from build123d import *

# Parameters (mm, degrees)
SKETCH_1_W             = 30
SKETCH_1_H             = 20
SKETCH_1_R             = 1.5
EXTRUDE_1_DEPTH        = 5
CUT_EXTRUDE_1_DEPTH    = 19.708286934
PATTERN_LINEAR_1_COUNT = 10
PATTERN_LINEAR_1_PITCH = 3


with BuildPart() as part:
    # 草图1 → 凸台-拉伸1 (new body)
    with BuildSketch(Plane(origin=(0, 0, 0), x_dir=(1, 0, 0), z_dir=(0, 1, 0))):
        Rectangle(SKETCH_1_W, SKETCH_1_H)
        with Locations(Location((-10, 7, 0), (0, 0, 270))):
            Circle(SKETCH_1_R, mode=Mode.SUBTRACT)
        with Locations(Location((10, 7, 0), (0, 0, 90))):
            Circle(SKETCH_1_R, mode=Mode.SUBTRACT)
        with Locations(Location((10, -7, 0), (0, 0, 270))):
            Circle(SKETCH_1_R, mode=Mode.SUBTRACT)
        with Locations(Location((-10, -7, 0), (0, 0, 90))):
            Circle(SKETCH_1_R, mode=Mode.SUBTRACT)
        with Locations(Location((0, 0, 0), (0, 0, 270))):
            Circle(SKETCH_1_R, mode=Mode.SUBTRACT)
    extrude(amount=EXTRUDE_1_DEPTH)

    # 草图2 → 切除-拉伸1 (cut, symmetric)
    with BuildSketch(Plane.XY):
        Polygon((-85.827625303, 0), (-15, 0), (-14.2, 0), (-13.5, 1.212435565), (-12.7, 1.212435565), (-12, 0), (23.413812651, -61.338522802), (-45.939949713, -184.854779506), (-155.181387668, -123.516256704), align=None)
    cut_extrude_1 = extrude(amount=CUT_EXTRUDE_1_DEPTH, both=True, mode=Mode.SUBTRACT)

    # 阵列(线性)1: 切除-拉伸1 ×10
    with Locations(*[(i * PATTERN_LINEAR_1_PITCH, 0, 0) for i in range(1, PATTERN_LINEAR_1_COUNT)]):
        add(cut_extrude_1, mode=Mode.SUBTRACT)


solid = part.part
Input: part model. Units: mm. Frame: model coordinates. A direction names the side the tool comes from. Coordinates: 2 decimals unless noted, no trailing zeros. Loops run counter-clockwise (first coordinate to the right, second up) from the corner with the lowest first, then second, coordinate; pieces in that order, holes last. Notation, with made-up numbers: (-9, 52) -> (48, 52) arc R16 cw to (48, 57) -> close; hole circle Ø10 at (38.5, -13.75). An arc over 180 degrees is marked (long way). One line per item, written item: value.
(1) Ray query, line 1 along X through (y, z) = (2.6, 7); line 2 along Z through (x, y) = (-10, 3.15); line 3 along X through (y, z) = (3.6, 0). Return the intervals inside material, ascending.
Answer below:
line 1: x = -15 to -11.5, -8.5 to 8.5, 11.5 to 15
line 2: z = -10 to -8.5, -5.5 to 5.5, 8.5 to 10
line 3: x = -15 to -1.5, 1.5 to 15
(2) Cut plane A-A (x = -10). Output: boundary loops of the cut face in (y, z), then the cut area to 3 significant figures.
Answer below:
outline: (1.21, -10) -> (5, -10) -> (5, -8.5) -> (1.21, -8.5) -> close; (1.21, -5.5) -> (5, -5.5) -> (5, 5.5) -> (1.21, 5.5) -> close; (1.21, 8.5) -> (5, 8.5) -> (5, 10) -> (1.21, 10) -> close
area: 53.0 mm2
(3) Cut plane D-D (x = 8). Output: boundary loops of the cut face in (y, z), then the cut area to 3 significant figures.
Answer below:
outline: (1.21, -10) -> (5, -10) -> (5, 10) -> (1.21, 10) -> close
area: 75.8 mm2
(4) Draft query along Z for faces 1 (the face through (8.513, 3.021, -6.805)), 2 (the face through (-4, 1.212, 0)). Return one class per face: pulls with the +Z half, pulls with the -Z half, needs draft (parallel to the pull), parting line crosses it, or undercut.
Answer below:
face 1: undercut
face 2: needs draft
(5) Cut plane C-C (z = 7). Give the number of separate pieces and of enclosed holes in the cut face, then the cut area to 3 significant figures.
Answer below:
separate pieces: 3
enclosed holes: 0
area: 105 mm2
(6) Pin query (flat end, axial travel): pin 1 Ø2.5 at (x, z) = (-10, 7) entering from -Y; pin 2 Ø4 at (x, z) = (-10, -7) entering from +Y; pin 3 Ø0.9 at (x, z) = (-4, 1) entering from -Y; pin 4 Ø0.9 at (x, z) = (1.5, 2.5) entering from -Y. Return the tip coordinate at first contact, or that it passes through.
Answer below:
pin 1: passes through
pin 2: stops at y = 5
pin 3: stops at y = 0.95
pin 4: stops at y = 0.43
(7) Set-up query: faces 3 (the face through (-8.6, 0, -0.1)), 4 (the face through (-10, 1.212, 9)). Return all of +Z, -Z, +X, -X, +Y, -Y with unobstructed straight access to the full face (end or side cutting, diameter ignored); none if empty.
Answer below:
face 3: +Z, -Z, +X, -X, -Y
face 4: +Z, -Z, -Y
(8) Cut plane B-B (y = 3.3). Output: boundary loops of the cut face in (x, z).
Answer below:
outline: (-15, -10) -> (15, -10) -> (15, 10) -> (-15, 10) -> close; hole circle Ø3 at (-10, -7); hole circle Ø3 at (-10, 7); hole circle Ø3 at (0, 0); hole circle Ø3 at (10, -7); hole circle Ø3 at (10, 7)
